For this review, take the finished solid that the model builds, in its own axes (mm). A direction names the side the tool comes from. Round coordinates to 2 decimals unless told otherwise and drop trailing zeros. Order: outer loops, then holes, each group sorted by start corner. A loop starts at its lowest first (then second) coordinate and runs counter-clockwise, first axis right, second up. Notation, with made-up numbers: M -14,29 L 25,29 A17 ccw 25,37 Z; hole C -15.5,37.5 d8. An arc over 180 degrees is marked long. Write item = value, one per line. Start each with the question number.
from build123d import *

# Parameters (mm, degrees)
F1_DEPTH  = 2
F0_W      = 6
F0_H      = 5.1
F2_DEPTH  = 1.1
F3_W      = 2.8
F3_H      = 0.2
F4_DEPTH  = 2
F5_R      = 1.25
F6_DEPTH  = 8.5
F7_R      = 0.75
F8_DEPTH  = 3
F9_R      = 0.9
F10_DEPTH = 7.7
F11_SIZE2 = 0.69282
F11_SIZE  = 1.2
F13_DEPTH = 12.5


with BuildPart() as f1:
    # F0 (on Front) → F1 (new body, symmetric)
    with BuildSketch(Plane.XZ):
        Polygon((-6, 5.1), (0, 5.1), (2.5, 5.1), (2.5, 9.7), (-0.9, 9.7), (-0.9, 13.7), (-1.6, 13.7), (-1.6, 9.9), (-2.2, 9.9), (-2.2, 13.7), (-2.9, 13.7), (-2.9, 9.7), (-6, 9.7), align=None)
    extrude(amount=F1_DEPTH, both=True)

    # F0 (on Front) → F2 (join, symmetric)
    with BuildSketch(Plane.XZ):
        with Locations((-3, 2.55)):
            Rectangle(F0_W, F0_H)
    extrude(amount=F2_DEPTH, both=True)

    # F3 (on face) → F4 (cut)
    with BuildSketch(Plane.YZ.offset(-0.9)):
        with Locations((0, 13.8)):
            Rectangle(F3_W, F3_H)
        with BuildLine():
            Line((-1.4, 13.7), (-1.4, 12.5))
            ThreePointArc((-1.4, 12.5), (0, 11.1), (1.4, 12.5))
            Line((1.4, 12.5), (1.4, 13.7))
            Line((1.4, 13.7), (-1.4, 13.7))
        make_face()
    extrude(amount=-F4_DEPTH, mode=Mode.SUBTRACT)

    # F5 (on face) → F6 (cut)
    with BuildSketch(Plane.YZ.offset(2.5)):
        with Locations((0, 6.7)):
            Circle(F5_R)
    extrude(amount=-F6_DEPTH, mode=Mode.SUBTRACT)

    # F7 (on face) → F8 (cut)
    with BuildSketch(Plane.XY.offset(9.7)):
        with Locations((0.4, 0)):
            Circle(F7_R)
    extrude(amount=-F8_DEPTH, mode=Mode.SUBTRACT)

    # F9 (on face) → F10 (cut)
    with BuildSketch(Plane.XY.offset(9.7)):
        with Locations((-4.6, 0)):
            Circle(F9_R)
    extrude(amount=-F10_DEPTH, mode=Mode.SUBTRACT)

    # F11
    f11_edges = [f1.edges().sort_by_distance(p)[0] for p in [
        (-3, -1.1, 0),
        (-3, 1.1, 0),
    ]]
    chamfer(f11_edges, length=F11_SIZE, length2=F11_SIZE2)

    # F12 (on Front) → F13 (cut, symmetric)
    with BuildSketch(Plane.XZ):
        Polygon((-2.511918, 0.011918), (-3, 0.5), (-3.488082, 0.011918), (-4.032431, 0.556267), (-4.478758, 0.109941), (-5.104953, 0.736136), (-5.5187, 0.322389), (-6, 0.803689), (-6, 0), (0, 0), (0, 0.803689), (-0.4813, 0.322389), (-0.895047, 0.736136), (-1.521242, 0.109941), (-1.967569, 0.556267), align=None)
    extrude(amount=F13_DEPTH, both=True, mode=Mode.SUBTRACT)


solid = f1.part
(1) For faces 1 (the flat face through (0, 0, 3)), 2 (the flat face through (-1.6, -0.5, 11)), 3 (the flat face through (-3, 1.1, 3)), 4 (the flat face through (-5, 0, 2)), list the 3-axis set-ups (+Z, -Z, +X, -X, +Y, -Y) from which the entire face can be reached by the end or side of a thin tool; tool diameter is ignored.
(2) We need section B-B, the plane y = 0. State how many separate pieces and enclosed holes the cut face has, then the cut area to 3 significant figures.
(3) We need section C-C, the plane z = 9. Write out the cut boundary in (x, y).
(4) Insertion check: pin 1 (1.2 mm diameter, centred on x = -3.5, z = 2, fed in from +Y); pin 2 (1.4 mm diameter, centred on x = -4.6, y = 0, fed in from +Z); pin 3 (1.1 mm diameter, centred on x = -4.6, y = 0, fed in from -Z). Each pin has a flat end and moves straight along its axis. Give the tip position at first contact, or say it passes through.
(5) For line 1 along X through (y, z) = (0, 9.3); line 2 along Y through (x, z) = (-4.6, 8.4); line 3 along Y through (x, z) = (-1, 12.75), list the stretches that pass through material, from the lowest coordinate up.
(6) Draft analysis for pull direction X (two halves, no side actions). For faces 5 (the flat face through (-0.9, 0, 10.8)), 6 (the cylindrical face through (-3.74, 0.27, 3.94)), 7 (the flat face through (-4, -1, 9.7)), state which applies: released by +X, released by -X, zero draft, split by the parting line, or undercut.
(7) We need section D-D, the plane z = 7. Write out the cut boundary in (x, y).
(8) We need section A-A, the plane x = 1.5. Write out the cut boundary in (y, z).
Values:
q1.face_1 = -Z, +X, +Y, -Y
q1.face_2 = +Z, +Y, -Y
q1.face_3 = -Z, +X, -X, +Y
q1.face_4 = +Z
q2.separate_pieces = 4
q2.enclosed_holes = 0
q2.area = 36.2 mm²
q3.outline = M -6,-2 L 2.5,-2 L 2.5,2 L -6,2 Z; hole C -4.6,0 d1.8; hole C 0.4,0 d1.5
q4.pin_1 = 1.1
q4.pin_2 = 2
q4.pin_3 = 0.11
q5.line_1 = -6 to -5.5, -3.7 to -0.35, 1.15 to 2.5
q5.line_2 = -2 to -0.9, 0.9 to 2
q5.line_3 = -2 to -1.4, 1.4 to 2
q6.face_5 = released by +X
q6.face_6 = undercut
q6.face_7 = zero draft
q7.outline = M -6,-2 L 2.5,-2 L 2.5,-1.21 L -6,-1.21 Z; M -6,1.21 L 2.5,1.21 L 2.5,2 L -6,2 Z
q8.outline = M -2,5.1 L 2,5.1 L 2,9.7 L -2,9.7 Z; hole C 0,6.7 d2.5
